Design review of the part built by this model. Coordinates are the model's own, in mm. Face numbers are marked on the shaded views. A direction names the side the tool comes from. Round coordinates to 2 decimals unless told otherwise and drop trailing zeros. Loops run counter-clockwise (first coordinate to the right, second up) from the corner with the lowest first, then second, coordinate; pieces in that order, holes last. Notation, with made-up numbers: (63, 57) - (109, 57) arc R31 cw to (109, 95) - close; hole circle Ø7 at (24.5, 59). An arc over 180 degrees is marked (long way). Use one line per item in the form item = value. Start each with the question number.
(1) For pin 1 (4 mm diameter, centred on x = -1, z = 15.5, fed in from +Y); pin 2 (0.6 mm diameter, centred on x = 0.5, y = -12.5, fed in from +Z); pin 3 (2 mm diameter, centred on x = 6, y = 9.5, fed in from +Z); pin 4 (3.5 mm diameter, centred on x = 1, z = -5, fed in from +Y), all flat-tipped, find the tip position at first contact; note any pin that passes through.
(2) We need section C-C, the plane z = 94.5. Write out the cut boundary in (x, y), then the cut area to 3 significant figures.
(3) Machinability: for the marked faces 1 and 2, which of the approach directions +Z, -Z, +X, -X, +Y, -Y give a long, thin tool a straight path to every point of the face, cutting with its end or side? Answer none if there is none.
(4) We need section B-B, the plane x = 0. Give the number of separate pieces and of enclosed holes in the cut face, then the cut area to 3 significant figures.
(5) Wall thickness on probe 1 along Y at (x, z) = (0, 20.25); probe 2 along Z at (x, y) = (-0.75, -0.25); probe 3 along Y at (x, z) = (0, 0): over which ranges is each line inside the solid? List them lowest first. Write a range as [from, to].
(6) We need section A-A, the plane z = 0. Write out the cut boundary in (x, y).
from build123d import *

# Parameters (mm, degrees)
BASE_EXTRUDE_DEPTH       = 4.1671875
SKETCH2_R                = 13.25
BOSS_EXTRUDE1_DEPTH      = 7.55
BOSS_EXTRUDE1_DEPTH_BACK = 7.55
SKETCH3_R                = 4.7625
SKETCH3_W                = 4.7625
SKETCH3_H                = 12.303125
CUT_EXTRUDE1_DEPTH       = 8.55
CUT_EXTRUDE1_DEPTH_BACK  = 8.55
SKETCH4_R                = 3.175
BOSS_EXTRUDE3_DEPTH      = 3.96875
SKETCH6_R                = 3.621484375
CUT_EXTRUDE2_DEPTH       = 3.96875
FILLET1_R                = 1
FILLET2_R                = 1
SKETCH7_W                = 4.365625
SKETCH7_H                = 1.537890625
CUT_EXTRUDE3_DEPTH       = 23.0265625
CUT_EXTRUDE3_DEPTH_BACK  = 15.0890625
BOSS_EXTRUDE4_START      = 1
SKETCH8_R                = 4.1671875
BOSS_EXTRUDE4_DEPTH      = 3.7625
SKETCH9_R                = 2.621484375
BOSS_EXTRUDE5_DEPTH      = 90
SKETCH10_R               = 4.1671875
BOSS_EXTRUDE6_DEPTH      = 5


with BuildPart() as part:
    # Sketch1 → Base-Extrude (new body, symmetric)
    with BuildSketch(Plane(origin=(0, 0, 0), x_dir=(0, 0, -1), z_dir=(1, 0, 0))):
        with BuildLine():
            Line((-10.41796875, 14.2875), (10.41796875, 14.2875))
            Line((10.41796875, 14.2875), (10.41796875, 9.485125685))
            ThreePointArc((10.41796875, 9.485125685), (14.0890625, 0), (10.41796875, -9.485125685))
            Line((10.41796875, -9.485125685), (10.41796875, -14.2875))
            Line((10.41796875, -14.2875), (-10.41796875, -14.2875))
            Line((-10.41796875, -14.2875), (-10.41796875, -10.41796875))
            Line((-10.41796875, -10.41796875), (-22.0265625, -10.41796875))
            Line((-22.0265625, -10.41796875), (-22.0265625, 10.41796875))
            Line((-22.0265625, 10.41796875), (-10.41796875, 10.41796875))
            Line((-10.41796875, 10.41796875), (-10.41796875, 14.2875))
        make_face()
    extrude(amount=BASE_EXTRUDE_DEPTH, both=True)

    # Sketch2 → Boss-Extrude1 (add, two sides)
    with BuildSketch(Plane(origin=(0, 0, 0), x_dir=(0, 0, -1), z_dir=(1, 0, 0))) as boss_extrude1_sk:
        Circle(SKETCH2_R)
    extrude(amount=BOSS_EXTRUDE1_DEPTH)
    extrude(boss_extrude1_sk.sketch, amount=-BOSS_EXTRUDE1_DEPTH_BACK)

    # Sketch3 → Cut-Extrude1 (cut, two sides)
    with BuildSketch(Plane(origin=(0, 0, 0), x_dir=(0, 0, -1), z_dir=(1, 0, 0))) as cut_extrude1_sk:
        Circle(SKETCH3_R)
        with Locations((-15.6765625, 0)):
            Rectangle(SKETCH3_W, SKETCH3_H)
    extrude(amount=CUT_EXTRUDE1_DEPTH, mode=Mode.SUBTRACT)
    extrude(cut_extrude1_sk.sketch, amount=-CUT_EXTRUDE1_DEPTH_BACK, mode=Mode.SUBTRACT)

    # Sketch4 → Boss-Extrude3 (add)
    with BuildSketch(Plane.XY.offset(22.0265625)):
        Circle(SKETCH4_R)
    extrude(amount=-BOSS_EXTRUDE3_DEPTH)

    # Sketch6 → Cut-Extrude2 (cut)
    with BuildSketch(Plane.XY.offset(22.0265625)):
        Circle(SKETCH6_R)
    extrude(amount=-CUT_EXTRUDE2_DEPTH, mode=Mode.SUBTRACT)

    # Fillet1
    fillet1_edges = [part.edges().sort_by_distance(p)[0] for p in [
        (0, 9.485125685, -10.41796875),
        (0, -9.485125685, -10.41796875),
        (0, -10.41796875, 10.41796875),
        (0, 10.41796875, 10.41796875),
    ]]
    fillet(fillet1_edges, radius=FILLET1_R)

    # Fillet2
    fillet2_edges = [part.edges().sort_by_distance(p)[0] for p in [
        (0, 14.2875, 10.41796875),
        (0, 14.2875, -10.41796875),
        (0, -14.2875, -10.41796875),
        (0, -14.2875, 10.41796875),
        (0, -10.41796875, 22.0265625),
        (0, 10.41796875, 22.0265625),
    ]]
    fillet(fillet2_edges, radius=FILLET2_R)

    # Sketch7 → Cut-Extrude3 (cut, two sides)
    with BuildSketch(Plane.XY) as cut_extrude3_sk:
        with Locations((0, 13.518554688)):
            Rectangle(SKETCH7_W, SKETCH7_H)
        with Locations((0, -13.518554688)):
            Rectangle(SKETCH7_W, SKETCH7_H)
    extrude(amount=CUT_EXTRUDE3_DEPTH, mode=Mode.SUBTRACT)
    extrude(cut_extrude3_sk.sketch, amount=-CUT_EXTRUDE3_DEPTH_BACK, mode=Mode.SUBTRACT)

    # Sketch8 → Boss-Extrude4 (add)
    with BuildSketch(Plane.XY.offset(13.2953125).offset(BOSS_EXTRUDE4_START)):
        Circle(SKETCH8_R)
    extrude(amount=BOSS_EXTRUDE4_DEPTH)

    # Sketch9 → Boss-Extrude5 (add)
    with BuildSketch(Plane.XY.offset(18.0578125)):
        Circle(SKETCH9_R)
    extrude(amount=BOSS_EXTRUDE5_DEPTH)

    # Sketch10 → Boss-Extrude6 (add)
    with BuildSketch(Plane.XY.offset(108.0578125)):
        Circle(SKETCH10_R)
    extrude(amount=BOSS_EXTRUDE6_DEPTH)


solid = part.part
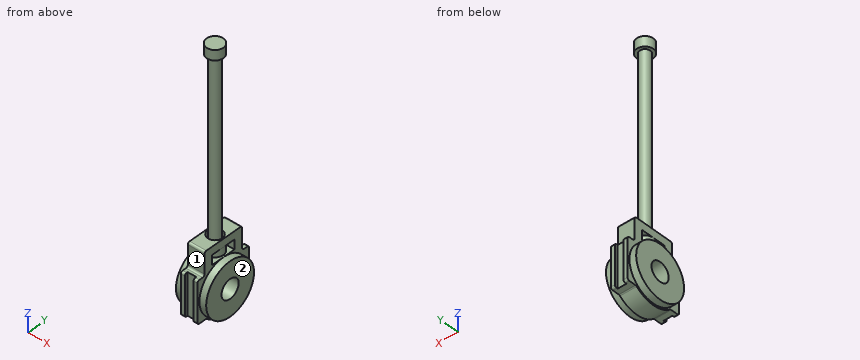
Data:
q1.pin_1 = 10.42
q1.pin_2 = 10.42
q1.pin_3 = 10.16
q1.pin_4 = 14.29
q2.outline = circle Ø5.24 at (0, 0)
q2.area = 21.6 mm^2
q3.face_1 = +Z, +X, -X, -Y
q3.face_2 = +Z, -Z, +X, +Y, -Y
q4.separate_pieces = 1
q4.enclosed_holes = 2
q4.area = 1,210 mm^2
q5.probe_1 = [-10.42, -3.62], [-2.62, 2.62], [3.62, 10.42]
q5.probe_2 = [-14.09, -4.76], [4.76, 13.3], [14.3, 113.06]
q5.probe_3 = [-12.75, -4.76], [4.76, 12.75]
q6.outline = (-7.55, -13.25) - (-4.17, -13.25) - (-4.17, -14.29) - (-2.18, -14.29) - (-2.18, -12.75) - (2.18, -12.75) - (2.18, -14.29) - (4.17, -14.29) - (4.17, -13.25) - (7.55, -13.25) - (7.55, -4.76) - (-7.55, -4.76) - close; (-7.55, 4.76) - (7.55, 4.76) - (7.55, 13.25) - (4.17, 13.25) - (4.17, 14.29) - (2.18, 14.29) - (2.18, 12.75) - (-2.18, 12.75) - (-2.18, 14.29) - (-4.17, 14.29) - (-4.17, 13.25) - (-7.55, 13.25) - close
